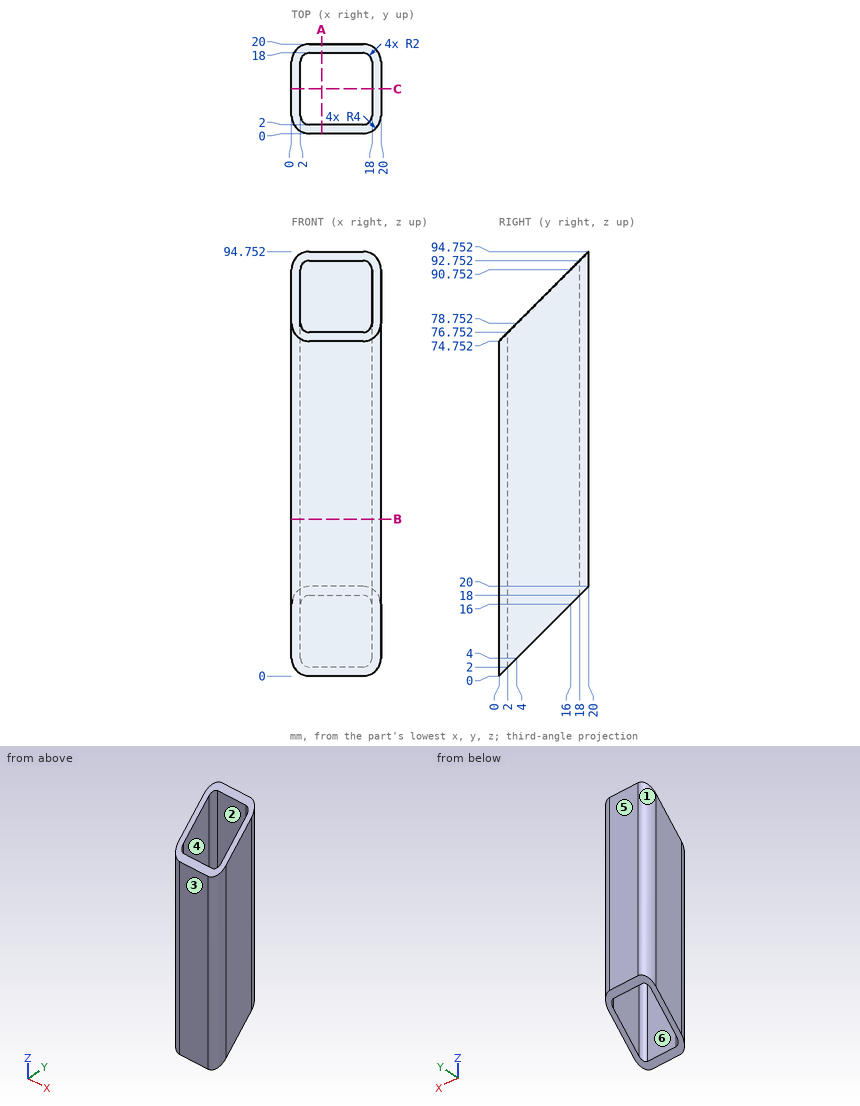
The figure shows three views and two pictorial views of one solid part (mm, origin at its lowest corner). Answer the questions. A direction names the side the tool comes from. Give positions to 0.01 mm unless a question says otherwise; leave off trailing zeros. Write each loop counter-clockwise with the first axis right and the second up, starting at its lowest first coordinate (ties: lowest second). Pieces come first, ordered by that corner, then holes.
Q1. The part is cut by section A-A on x = 6.75. Give the vertices of the cut face in (y, z), and give its area (3 significant figures).
Answer:
outline: (0, 0) - (2, 2) - (2, 76.75) - (0, 74.75) - close; (18, 18) - (20, 20) - (20, 94.75) - (18, 92.75) - close
area: 299 mm2
Q2. Given pin 1 (4 mm diameter, centred on x = 2.5, y = 7, fed in from -Z); pin 2 (1 mm diameter, centred on x = 12.5, z = 16, fed in from +Y), each flat-ended and moving along its own axis, determine where each tip first touches the part or whether it passes through.
Answer:
pin 1: stops at z = 5.06
pin 2: stops at y = 2
Q3. A tool of negligible diameter and unlimited length cuts with its end or side. For the marked faces 5 and 6, from which of +Z, -Z, +X, -X, +Y, -Y can it reach the whole face along a straight path? Write none if from no direction.
Answer:
face 5: +Z, -Z, +X, -X, +Y
face 6: +Z, -Z
Q4. Straight lines are drawn through the part: L1, parallel to Y at x = 16, z = 38.5; L2, parallel to Y at x = 10.25, z = 91. For each, find the intervals that lie inside material, in ascending order.
Answer:
L1: y = 0 to 2, 18 to 20
L2: y = 18 to 20
Q5. The part is cut by section B-B on z = 35. Give the vertices of the cut face in (x, y), and give its area (3 significant figures).
Answer:
outline: (0, 4) arc R4 ccw to (4, 0) - (16, 0) arc R4 ccw to (20, 4) - (20, 16) arc R4 ccw to (16, 20) - (4, 20) arc R4 ccw to (0, 16) - close; hole (2, 4) arc R2 ccw to (4, 2) - (16, 2) arc R2 ccw to (18, 4) - (18, 16) arc R2 ccw to (16, 18) - (4, 18) arc R2 ccw to (2, 16) - close
area: 134 mm2
Q6. For a pull along Y with two mould halves and no side action, classify the marked faces 1, 2, 3 and 4 as released by +Y, released by -Y, zero draft, split by the parting line, or undercut.
Answer:
face 1: released by +Y
face 2: undercut
face 3: released by -Y
face 4: undercut
Q7. The part is cut by section C-C on y = 10. Give the vertices of the cut face in (x, z).
Answer:
outline: (0, 10) - (2, 10) - (2, 84.75) - (0, 84.75) - close; (18, 10) - (20, 10) - (20, 84.75) - (18, 84.75) - close
